The model under review builds one solid part; all positions refer to its coordinate system, in mm. A direction names the side the tool comes from. Give positions to 0.01 mm unless a question says otherwise; leave off trailing zeros. Order: outer loops, then holes, each group sorted by start corner. A loop starts at its lowest first (then second) coordinate and runs counter-clockwise, first axis right, second up.
```python
from build123d import *

# Parameters (mm, degrees)
SKETCH2_R               = 11.05
BOSS_EXTRUDE1_DEPTH     = 9
CHAMFER1_SIZE           = 8
SKETCH3_R               = 13
SKETCH3_R_2             = 10
BOSS_EXTRUDE2_DEPTH     = 2
SKETCH5_W               = 56
SKETCH5_H               = 11
BOSS_EXTRUDE3_DEPTH     = 5
SKETCH6_R               = 2.55
CUT_EXTRUDE5_DEPTH      = 47.989360498
CUT_EXTRUDE6_DEPTH      = 10
CUT_EXTRUDE6_DEPTH_BACK = 1.5
SKETCH7_R               = 5
FILLET1_R               = 6


with BuildPart() as part:
    # Sketch2 → Boss-Extrude1 (new body)
    with BuildSketch(Plane(origin=(0, 0, 0), x_dir=(1, 0, 0), z_dir=(0, 1, 0))):
        Polygon((-28, 21), (28, 21), (28, 16), (16, 16), (16, -16), (-16, -16), (-16, 16), (-28, 16), align=None)
        with Locations(Location((0, 0, 0), (0, 0, 270))):
            Circle(SKETCH2_R, mode=Mode.SUBTRACT)
    extrude(amount=BOSS_EXTRUDE1_DEPTH)

    # Chamfer1
    chamfer1_edges = [part.edges().sort_by_distance(p)[0] for p in [
        (16, 4.5, 16),
        (-16, 4.5, 16),
    ]]
    chamfer(chamfer1_edges, length=CHAMFER1_SIZE)

    # Sketch3 → Boss-Extrude2 (add)
    with BuildSketch(Plane.XZ):
        Circle(SKETCH3_R)
        with Locations(Location((0, 0, 0), (0, 0, 270))):
            Circle(SKETCH3_R_2, mode=Mode.SUBTRACT)
    extrude(amount=-BOSS_EXTRUDE2_DEPTH)

    # Sketch5 → Boss-Extrude3 (add)
    with BuildSketch(Plane.XY.offset(-16)):
        with Locations((0, 14.5)):
            Rectangle(SKETCH5_W, SKETCH5_H)
    extrude(amount=-BOSS_EXTRUDE3_DEPTH)

    # Sketch6 → Cut-Extrude5 (cut, through all)
    with BuildSketch(Plane.XY.offset(-16)):
        with Locations((-22, 10)):
            Circle(SKETCH6_R)
        with Locations((22, 10.340473159)):
            Circle(SKETCH6_R)
    extrude(amount=-CUT_EXTRUDE5_DEPTH, mode=Mode.SUBTRACT)

    # Sketch7 → Cut-Extrude6 (cut, two sides: drawn at the far end of the back side and taken through both)
    with BuildSketch(Plane.XY.offset(-16).offset(-CUT_EXTRUDE6_DEPTH_BACK)):
        with Locations(Location((22, 10.340473159, 0), (0, 0, 180))):
            Circle(SKETCH7_R)
        with Locations(Location((-22, 10, 0), (0, 0, 180))):
            Circle(SKETCH7_R)
    extrude(amount=CUT_EXTRUDE6_DEPTH + CUT_EXTRUDE6_DEPTH_BACK, mode=Mode.SUBTRACT)

    # Fillet1
    # the kernel refuses this fillet: 6 mm, written as the material it adds along each edge
    with BuildSketch(Plane(origin=(-16, 0, -16), x_dir=(-1, 0, 0), z_dir=(0, 1, 0))) as fillet1_piece_1_section:
        with BuildLine():
            CenterArc((FILLET1_R, FILLET1_R), FILLET1_R, 180, 90)
            Line((0, FILLET1_R), (0, 0))
            Line((0, 0), (FILLET1_R, 0))
        make_face()
    fillet1_piece_1 = extrude(amount=9, mode=Mode.PRIVATE)
    fillet1_piece_1 = fillet1_piece_1 - Plane(origin=(-22, 10, -14.524998949), x_dir=(-1, 0, 0), z_dir=(0, 0, 1)) * Cylinder(5, 43, mode=Mode.PRIVATE)
    add(fillet1_piece_1)
    with BuildSketch(Plane(origin=(16, 0, -16), x_dir=(0, 0, 1), z_dir=(0, 1, 0))) as fillet1_piece_2_section:
        with BuildLine():
            CenterArc((FILLET1_R, FILLET1_R), FILLET1_R, 180, 90)
            Line((0, FILLET1_R), (0, 0))
            Line((0, 0), (FILLET1_R, 0))
        make_face()
    fillet1_piece_2 = extrude(amount=9, mode=Mode.PRIVATE)
    fillet1_piece_2 = fillet1_piece_2 - Plane(origin=(22, 10.340473159, -14.541701279), x_dir=(-1, 0, 0), z_dir=(0, 0, 1)) * Cylinder(5, 42, mode=Mode.PRIVATE)
    add(fillet1_piece_2)
    # the kernel refuses this fillet: 6 mm, written as the material it takes off along each edge
    with BuildSketch(Plane(origin=(16, -6.213203436, 8), x_dir=(0, 0, -1), z_dir=(0, 1, 0))) as fillet1_2_piece_1:
        with BuildLine():
            CenterArc((FILLET1_R * 0.414213562373, FILLET1_R), FILLET1_R, 225, 45)
            Line((-FILLET1_R * 0.292893218813, FILLET1_R * 0.292893218813), (0, 0))
            Line((0, 0), (FILLET1_R * 0.414213562373, 0))
        make_face()
    extrude(amount=21.426406871, mode=Mode.SUBTRACT)
    with BuildSketch(Plane(origin=(8, -6.213203436, 16), x_dir=(-1, 0, 0), z_dir=(0, 1, 0)), Plane(origin=(-8, -6.213203436, 16), x_dir=(-0.7071067811865481, 0, -0.707106781186547), z_dir=(0, 1, 0)), Plane(origin=(-16, -6.213203436, 8), x_dir=(0, 0, -1), z_dir=(0, 1, 0))) as fillet1_2_piece_2:
        with BuildLine():
            CenterArc((FILLET1_R * 0.414213562373, -FILLET1_R), FILLET1_R, 90, 45)
            Line((-FILLET1_R * 0.292893218813, -FILLET1_R * 0.292893218813), (0, 0))
            Line((0, 0), (FILLET1_R * 0.414213562373, 0))
        make_face()
    extrude(amount=21.426406871, mode=Mode.SUBTRACT)
    with BuildSketch(Plane(origin=(28, 0, -36), x_dir=(0, 1, 0), z_dir=(0, 0, 1)), Plane(origin=(28, 20, -1), x_dir=(0, -1, 0), z_dir=(0, 0, -1)), Plane(origin=(-28, 20, -1), x_dir=(1, 0, 0), z_dir=(0, 0, -1)), Plane(origin=(-28, 0, -1), x_dir=(0, 1, 0), z_dir=(0, 0, -1))) as fillet1_2_piece_3:
        with BuildLine():
            CenterArc((FILLET1_R, FILLET1_R), FILLET1_R, 180, 90)
            Line((0, FILLET1_R), (0, 0))
            Line((0, 0), (FILLET1_R, 0))
        make_face()
    extrude(amount=35, mode=Mode.SUBTRACT)


solid = part.part
```
1. Take a section at D-D (z = 4.5). Write out the cut boundary in (x, y).
2. For faces 4 (the cylindrical face through (-10.787, 5.451, -2.395)), 5 (the cylindrical face through (19.976, 8.789, -19.226)), 6 (the flat face through (16, 4, -2)), list the 3-axis set-ups (+Z, -Z, +X, -X, +Y, -Y) from which the entire face can be reached by the end or side of a thin tool; tool diameter is ignored.
3. Take a section at B-B (x = 0). Write out the cut boundary in (y, z).
4. To check wall thickness, follow line 1 (X direction, y = 10, z = -16.9); line 2 (X direction, y = 4, z = 0.5); line 3 (Z direction, x = 19, y = 12). State the ranges of each line that lie inside material, in increasing order.
5. Take a section at C-C (x = -12.5). Write out the cut boundary in (y, z).
6. Draft analysis for pull direction Y (two halves, no side actions). For faces 1 (the flat face through (-24, 12, -17.5)), 2 (the flat face through (-16, 4, -2)), 3 (the cylindrical face through (-26.196, 1.711, -18.465)), state which applies: pulls with the +Y half, pulls with the -Y half, needs draft (parallel to the pull), parting line crosses it, or undercut.
7. Insertion check: pin 1 (10 mm diameter, centred on y = 5, z = -0.5, fed in from -X); pin 2 (8 mm diameter, centred on x = -21.5, y = 11.5, fed in from +Z); pin 3 (10 mm diameter, centred on x = 14, y = 8.5, fed in from +Z). Each pin has a flat end and moves straight along its axis. Give the tip position at first contact, or say it passes through.
8. Take a section at A-A (z = 0). Write out the cut boundary in (x, y), and give its area (3 significant figures).
Answer:
1. outline: (-16, 0) - (-8.93, 0) - (-8.93, 2) - (-10.09, 2) - (-10.09, 9) - (-16, 9) - close; (8.93, 0) - (16, 0) - (16, 9) - (10.09, 9) - (10.09, 2) - (8.93, 2) - close
2. face 4: +Y
2. face 5: +Z, -Z
2. face 6: +Z, +X, +Y, -Y
3. outline: (0, -21) - (20, -21) - (20, -16) - (9, -16) - (9, -11.05) - (2, -11.05) - (2, -10) - (0, -10) - close; (0, 10) - (2, 10) - (2, 11.05) - (9, 11.05) - (9, 16) - (0, 16) - close
4. line 1: x = -28 to -27, -17 to 17.01, 26.99 to 28
4. line 2: x = -16 to -11.04, 11.04 to 16
4. line 3: z = -21 to -17.5
5. outline: (0, -21) - (20, -21) - (20, -16) - (9, -16) - (9, 11.5) - (0, 11.5) - close
6. face 1: undercut
6. face 2: needs draft
6. face 3: pulls with the -Y half
7. pin 1: stops at x = -16
7. pin 2: stops at z = -16
7. pin 3: stops at z = 14.88
8. outline: (-16, 0) - (-10, 0) - (-10, 2) - (-11.05, 2) - (-11.05, 9) - (-16, 9) - close; (10, 0) - (16, 0) - (16, 9) - (11.05, 9) - (11.05, 2) - (10, 2) - close
8. area: 93.3 mm2
